Check sheet for the modelled part. Datum: model origin and axes. Units: mm. Face numbers are marked on the shaded views. A direction names the side the tool comes from. Round coordinates to 2 decimals unless told otherwise and drop trailing zeros. Loops run counter-clockwise (first coordinate to the right, second up) from the corner with the lowest first, then second, coordinate; pieces in that order, holes last. Notation, with made-up numbers: (19, 19) - (34, 19) arc R14 ccw to (34, 27) - close; hole circle Ø2 at (-17, 89.5). An arc over 180 degrees is marked (long way). Return JSON: item names as keys, results as strings.
from build123d import *

# Parameters (mm, degrees)
SKETCH1_R                = 8.15
BOSS_EXTRUDE1_DEPTH      = 7
BOSS_EXTRUDE1_DEPTH_BACK = 7
CUT_EXTRUDE1_REACH       = 34
SKETCH2_R                = 1.75
FILLET1_R                = 10
SKETCH3_R                = 8.998813241
SKETCH3_R_2              = 5
BOSS_EXTRUDE2_DEPTH      = 4
CUT_EXTRUDE2_REACH       = 28
SKETCH4_R                = 4


with BuildPart() as part:
    # Sketch1 → Boss-Extrude1 (new body, two sides)
    with BuildSketch(Plane(origin=(0, 0, 0), x_dir=(1, 0, 0), z_dir=(0, 1, 0))) as boss_extrude1_sk:
        Polygon((-19, 0), (19, 0), (19, 6), (12, 6), (12, 32), (-12, 32), (-12, 6), (-19, 6), align=None)
        with Locations((0, 20)):
            Circle(SKETCH1_R, mode=Mode.SUBTRACT)
    extrude(amount=BOSS_EXTRUDE1_DEPTH)
    extrude(boss_extrude1_sk.sketch, amount=-BOSS_EXTRUDE1_DEPTH_BACK)

    # Sketch2 → Cut-Extrude1 (cut, up to next)
    with BuildSketch(Plane.XY, mode=Mode.PRIVATE) as cut_extrude1_sk1:
        with Locations((-15, 0)):
            Circle(SKETCH2_R)
    cut_extrude1_tool1 = extrude(cut_extrude1_sk1.sketch, amount=-CUT_EXTRUDE1_REACH, mode=Mode.PRIVATE) & part.part
    add(cut_extrude1_tool1.solids().sort_by_distance((-15, 0, 0))[0], mode=Mode.SUBTRACT)
    # Sketch2 → Cut-Extrude1 (cut, up to next)
    with BuildSketch(Plane.XY, mode=Mode.PRIVATE) as cut_extrude1_sk2:
        with Locations((15, 0)):
            Circle(SKETCH2_R)
    cut_extrude1_tool2 = extrude(cut_extrude1_sk2.sketch, amount=-CUT_EXTRUDE1_REACH, mode=Mode.PRIVATE) & part.part
    add(cut_extrude1_tool2.solids().sort_by_distance((15, 0, 0))[0], mode=Mode.SUBTRACT)

    # Fillet1
    fillet1_edges = [part.edges().sort_by_distance(p)[0] for p in [
        (-12, 0, -32),
        (12, 0, -32),
    ]]
    fillet(fillet1_edges, radius=FILLET1_R)

    # Sketch3 → Boss-Extrude2 (add)
    with BuildSketch(Plane(origin=(0, 7, 0), x_dir=(1, 0, 0), z_dir=(0, 1, 0))):
        with Locations((0, 20)):
            Circle(SKETCH3_R)
        with Locations((0, 20)):
            Circle(SKETCH3_R_2, mode=Mode.SUBTRACT)
    extrude(amount=-BOSS_EXTRUDE2_DEPTH)

    # Sketch4 → Cut-Extrude2 (cut, up to next)
    with BuildSketch(Plane(origin=(0, 0, -6), x_dir=(-1, 0, 0), z_dir=(0, 0, -1)), mode=Mode.PRIVATE) as cut_extrude2_sk1:
        with Locations((15, 0)):
            Circle(SKETCH4_R)
    cut_extrude2_tool1 = extrude(cut_extrude2_sk1.sketch, amount=CUT_EXTRUDE2_REACH, mode=Mode.PRIVATE) & part.part
    add(cut_extrude2_tool1.solids().sort_by_distance((-15, 0, -6))[0], mode=Mode.SUBTRACT)
    # Sketch4 → Cut-Extrude2 (cut, up to next)
    with BuildSketch(Plane(origin=(0, 0, -6), x_dir=(-1, 0, 0), z_dir=(0, 0, -1)), mode=Mode.PRIVATE) as cut_extrude2_sk2:
        with Locations((-15, 0)):
            Circle(SKETCH4_R)
    cut_extrude2_tool2 = extrude(cut_extrude2_sk2.sketch, amount=CUT_EXTRUDE2_REACH, mode=Mode.PRIVATE) & part.part
    add(cut_extrude2_tool2.solids().sort_by_distance((15, 0, -6))[0], mode=Mode.SUBTRACT)


solid = part.part
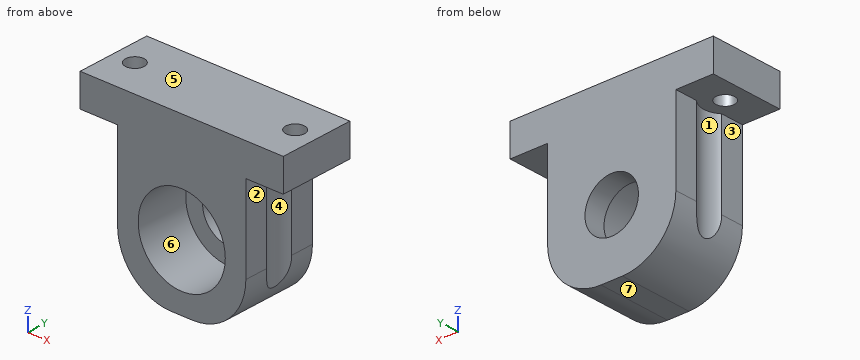
Q1. Sectioned sample at D-D (z = -3). Enter the section's corners in (x, y), plus the area to 3 significant figures.
Answer key:
{"outline": "(-19, -7) - (19, -7) - (19, 7) - (-19, 7) - close; hole circle Ø3.5 at (-15, 0); hole circle Ø3.5 at (15, 0)", "area": "513 mm²"}
Q2. Sectioned sample at C-C (x = -15). Enter the section's corners in (y, z), plus the area to 3 significant figures.
Answer key:
{"outline": "(-7, -6) - (-1.75, -6) - (-1.75, 0) - (-7, 0) - close; (1.75, -6) - (7, -6) - (7, 0) - (1.75, 0) - close", "area": "63.0 mm²"}
Q3. Tool access check on the marked faces 1, 2, 3 and 4. Record the directions out of +Z, -Z, +X, -X, +Y, -Y that give a thin tool (end or side, any length) a straight path to the whole face; none if there is none.
Answer key:
{"face 1": "-Z, -X", "face 2": "-Z, +X, +Y, -Y", "face 3": "-Z, -X, +Y, -Y", "face 4": "-Z, +X"}
Q4. Sectioned sample at A-A (y = 0). Enter the section's corners in (x, z), plus the area to 3 significant figures.
Answer key:
{"outline": "(-19, -6) - (-16.75, -6) - (-16.75, 0) - (-19, 0) - close; (-13.25, -6) - (-11, -6) - (-11, -26.36) arc R10 ccw to (-2, -32) - (2, -32) arc R10 ccw to (11, -26.36) - (11, -6) - (13.25, -6) - (13.25, 0) - (-13.25, 0) - close; (16.75, -6) - (19, -6) - (19, 0) - (16.75, 0) - close; hole circle Ø16.3 at (0, -20)", "area": "521 mm²"}
Q5. Depth check by flat-ended pin: P1, Ø8, axis at x = -3.5, y = 4, coming from the +Z side; P2, Ø4, axis at y = -4, z = -27, coming from the +X side; P3, Ø2, axis at y = -4, z = -11.5, coming from the +X side; P4, Ø1.5, axis at y = -3.5, z = -21, coming from the -X side. Enter the tip coordinate at first touch or a pass-through.
Answer key:
{"P1": "stops at z = 0", "P2": "stops at x = 11.54", "P3": "stops at x = 12", "P4": "stops at x = -12"}
Q6. Draft check along Z on the marked faces 5, 6 and 7. Enter one of: released by +Z, released by -Z, zero draft, split by the parting line, or undercut.
Answer key:
{"face 5": "released by +Z", "face 6": "undercut", "face 7": "released by -Z"}
Q7. Scan lines: probe 1 along Y at (x, z) = (15, -2); probe 2 along Z at (x, y) = (0, 6.1); probe 3 along Z at (x, y) = (0, -2.5). Record each from-to range of solid material in increasing order. Write a range as [from, to].
Answer key:
{"probe 1": "y = [-7, -1.75], [1.75, 7]", "probe 2": "z = [-32, -25], [-15, 0]", "probe 3": "z = [-32, -28.15], [-11.85, 0]"}
Q8. Sectioned sample at B-B (z = -20). Enter the section's corners in (x, y).
Answer key:
{"outline": "(-12, -7) - (-8.15, -7) - (-8.15, 3) - (-5, 3) - (-5, 7) - (-12, 7) - (-12, 2.65) arc R4 cw to (-12, -2.65) - close; (5, 3) - (8.15, 3) - (8.15, -7) - (12, -7) - (12, -2.65) arc R4 cw to (12, 2.65) - (12, 7) - (5, 7) - close"}
